Work out the finished part from the listing and answer in its coordinate system (mm). Face numbers are marked on the shaded views. Give positions to 0.01 mm unless a question says otherwise; leave off trailing zeros. Write each loop counter-clockwise with the first axis right and the second up, starting at its lowest first coordinate (ties: lowest second). Pieces come first, ordered by that corner, then holes. Notation, with made-up numbers: (-18, 27) - (36, 27) arc R17 ccw to (36, 31) - close; hole circle Ø5 at (-4, 63). An arc over 180 degrees is marked (long way). Write each question's results on one line, items separated by ' | '. Start each with the question number.
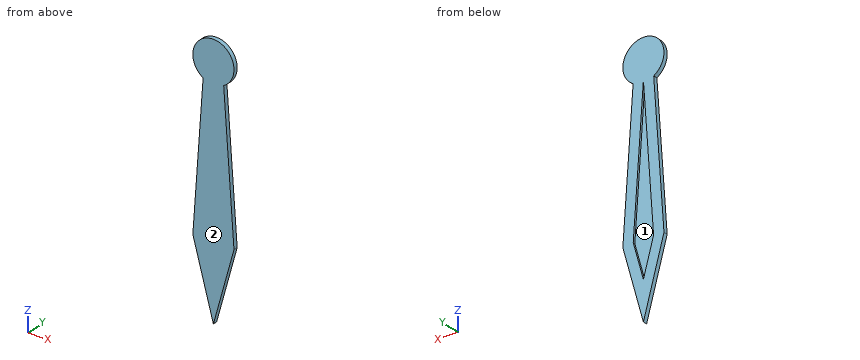
from build123d import *

# Parameters (mm, degrees)
EXTRUDE1_DEPTH = 0.2
EXTRUDE2_DEPTH = 0.1


with BuildPart() as part:
    # Sketch1 → Extrude1 (new body)
    with BuildSketch(Plane(origin=(0, 0, 0), x_dir=(1, 0, 0), z_dir=(0, 1, 0))):
        with BuildLine():
            Line((0, 11.5), (1, 7.9))
            Line((1, 7.9), (0.5, 0.866025404))
            ThreePointArc((0.5, 0.866025404), (0, -1), (-0.5, 0.866025404))
            Line((-0.5, 0.866025404), (-1, 7.9))
            Line((-1, 7.9), (0, 11.5))
        make_face()
    extrude(amount=EXTRUDE1_DEPTH)

    # Sketch2 → Extrude2 (cut)
    with BuildSketch(Plane(origin=(0, 0.2, 0), x_dir=(1, 0, 0), z_dir=(0, 1, 0))):
        Polygon((-0.001258451, 0.901477732), (0.001258451, 0.901477732), (0.495137938, 7.849349255), (0, 9.631845831), (-0.495137938, 7.849349255), align=None)
    extrude(amount=-EXTRUDE2_DEPTH, mode=Mode.SUBTRACT)


solid = part.part
Q1. A cutting plane is placed at A-A, the plane x = 0.85. Write down the section's boundary in (y, z).
Q2. A cutting plane is placed at D-D, the plane x = 0.15. Write down the section's boundary in (y, z), and give its area (3 significant figures).
Q3. Consider L1, parallel to X at y = 0.15, z = -4; L2, parallel to X at y = 0.1, z = -10.5. Determine where each line is inside the solid, lowest interval first.
Q4. A cutting plane is placed at C-C, the plane z = -2. Write down the section's boundary in (x, y), and give its area (3 significant figures).
Q5. The mould has two halves that part along X. Classify the marked faces 1 and 2: pulls with the +X half, pulls with the -X half, needs draft (parallel to the pull), parting line crosses it, or undercut.
Result:
1) outline: (0, -8.44) - (0.2, -8.44) - (0.2, -5.79) - (0, -5.79) - close; (0, -0.53) - (0.2, -0.53) - (0.2, 0.53) - (0, 0.53) - close
2) outline: (0, -10.96) - (0.2, -10.96) - (0.2, -9.09) - (0.1, -9.09) - (0.1, -2.99) - (0.2, -2.99) - (0.2, 0.99) - (0, 0.99) - close | area: 1.78 mm2
3) L1: x = -0.72 to -0.22, 0.22 to 0.72 | L2: x = -0.28 to 0.28
4) outline: (-0.58, 0) - (0.58, 0) - (0.58, 0.2) - (0.08, 0.2) - (0.08, 0.1) - (-0.08, 0.1) - (-0.08, 0.2) - (-0.58, 0.2) - close | area: 0.216 mm2
5) face 1: undercut | face 2: needs draft
